Check sheet for the modelled part. Datum: model origin and axes. Units: mm. Face numbers are marked on the shaded views. A direction names the side the tool comes from. Round coordinates to 2 decimals unless told otherwise and drop trailing zeros. Loops run counter-clockwise (first coordinate to the right, second up) from the corner with the lowest first, then second, coordinate; pieces in that order, holes last. Notation, with made-up numbers: (-13.75, 16) - (35.25, 16) arc R29 cw to (35.25, 53) - close; hole circle Ø11 at (-4.5, -20). An arc over 180 degrees is marked (long way). Put each result on its own line as item: value. Start each with the question number.
Item 1: Section check C-C, the plane y = 2.5. Record the cut outline in (x, z) (3 decimals).
Item 2: Material ranges on line 1 along Z through (x, y) = (1.5, 2.25) (3 decimals); line 2 along Y through (x, z) = (0, 7.45); line 3 along X through (y, z) = (-0.5, 1.5), recorded low to high.
Item 3: Section check B-B, the plane z = 7.75. Record the cut outline in (x, y) (1 decimal).
Item 4: Tool access check on the marked faces 1, 2 and 3. Record the directions out of +Z, -Z, +X, -X, +Y, -Y that give a thin tool (end or side, any length) a straight path to the whole face; none if there is none.
Item 5: Section check D-D, the plane x = 0.5. Give the number of separate pieces and of enclosed holes in the cut face, and give its area (3 significant figures).
Item 6: Gauge pin test, flat end, axial feed: pin 1 Ø2 at (x, z) = (-2, 1.5) entering from +Y. Record the tip position at first contact, or that the pin passes through.
Item 7: Draft check along X on the marked faces 4, 5 and 6. Enter one of: pulls with the +X half, pulls with the -X half, needs draft (parallel to the pull), parting line crosses it, or undercut.
from build123d import *

# Parameters (mm, degrees)
F0_R      = 1.5875
F1_DEPTH  = 3.175
F2_R      = 3.175
F3_DEPTH  = 3.175
F4_R      = 1.5875
F5_DEPTH  = 3.175
F6_T      = -0.254
F7_DEPTH  = 0.254
F8_SIZE   = 0.25399
F10_DEPTH = 4.175


# Not quite as in the source:
# - a fillet or chamfer is up to 0.001 mm smaller than in the source, because OpenCascade refuses the exact size


with BuildPart() as f1:
    # F0 (on Top) → F1 (new body)
    with BuildSketch(Plane.XY):
        Circle(F0_R)
    extrude(amount=F1_DEPTH)

    # F2 (on face) → F3 (join)
    with BuildSketch(Plane.XY.offset(3.175)):
        Circle(F2_R)
    extrude(amount=F3_DEPTH)

    # F4 (on face) → F5 (join)
    with BuildSketch(Plane.XY.offset(6.35)):
        Circle(F4_R)
    extrude(amount=F5_DEPTH)

    # F6
    f6_openings = [f1.faces().sort_by_distance(p)[0] for p in [
        (0, 0, 9.525),
    ]]
    offset(amount=F6_T, openings=f6_openings, kind=Kind.INTERSECTION)

    # F7 (cut, through all): a face of the model
    f7_faces = [f1.faces().sort_by_distance(p)[0] for p in [
        (0, 0, 0.254),
    ]]
    extrude(f7_faces, amount=-F7_DEPTH, mode=Mode.SUBTRACT)

    # F8 (size 0.254 in the source; OpenCascade refuses exactly that, so slightly less here)
    f8_edges = [f1.edges().sort_by_distance(p)[0] for p in [
        (-1.5875, 0, 9.525),
        (-1.5875, 0, 0),
    ]]
    chamfer(f8_edges, length=F8_SIZE)

    # F9 (on Front) → F10 (cut, up to face)
    with BuildSketch(Plane.XZ):
        Polygon((1.0448596497, 5.36575), (-1.0448596497, 5.36575), (0, 3.556), align=None)
    extrude(amount=-F10_DEPTH, mode=Mode.SUBTRACT)


solid = f1.part
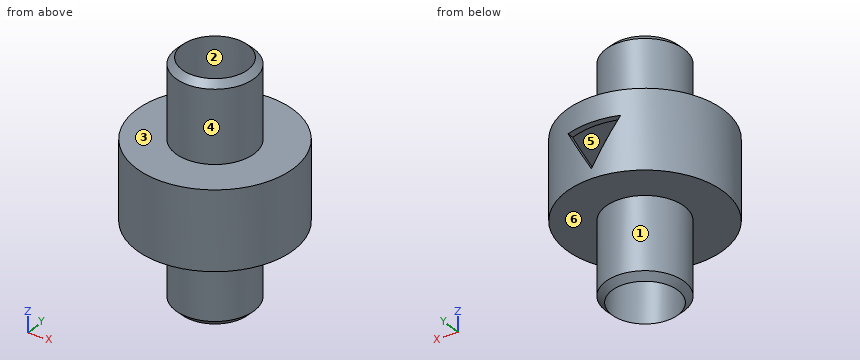
Check result:
1. outline: (-1.957, 3.175) - (1.957, 3.175) - (1.957, 6.35) - (-1.957, 6.35) - close; hole (-1.511, 3.429) - (1.511, 3.429) - (1.511, 6.096) - (-1.511, 6.096) - close
2. line 1: 3.175 to 3.429, 6.096 to 6.35
2. line 2: -1.59 to -1.33, 1.33 to 1.59
2. line 3: -1.51 to -1.24, 1.24 to 1.51
3. outline: circle Ø3.2 at (0, 0); hole circle Ø2.7 at (0, 0)
4. face 1: -Z
4. face 2: +Z, -Z
4. face 3: +Z
5. separate pieces: 3
5. enclosed holes: 0
5. area: 6.36 mm²
6. pin 1: y = 1.23
7. face 4: parting line crosses it
7. face 5: undercut
7. face 6: needs draft
